Source: CAD feature listing. Evaluate the final solid. Frame: model axes, mm. Give positions to 0.01 mm unless a question says otherwise; leave off trailing zeros. Loops run counter-clockwise (first coordinate to the right, second up) from the corner with the lowest first, then second, coordinate; pieces in that order, holes last. Notation, with made-up numbers: M 74,72 L 90,72 A25 cw 90,97 Z; hole C 17.25,-5.5 d4. An arc over 180 degrees is marked long. Write item = value, one per line.
from build123d import *

# Parameters (mm, degrees)
BOSS_EXTRUDE2_DEPTH = 4
SKETCH2_R           = 3.5
CUT_EXTRUDE1_DEPTH  = 4
SKETCH3_W           = 225
SKETCH3_H           = 150
BOSS_EXTRUDE3_DEPTH = 4


with BuildPart() as part:
    # Sketch1 → Boss-Extrude2 (new body)
    with BuildSketch(Plane(origin=(0, 0, 0), x_dir=(1, 0, 0), z_dir=(0, 1, 0))):
        Polygon((-120, 117), (-120, 150), (-135, 150), (-180, 0), (-135, 0), (0, 0), (45, 0), (0, 150), (-15, 150), (-15, 117), (-30, 117), (-30, 84), (-45, 84), (-45, 51), (-90, 51), (-90, 84), (-105, 84), (-105, 117), align=None)
    extrude(amount=BOSS_EXTRUDE2_DEPTH)

    # Sketch2 → Cut-Extrude1 (cut)
    with BuildSketch(Plane(origin=(0, 4, 0), x_dir=(1, 0, 0), z_dir=(0, 1, 0))):
        with Locations(Location((-127.5, 135, 0), (0, 0, 270))):
            Circle(SKETCH2_R)
        with Locations(Location((-112.5, 102, 0), (0, 0, 270))):
            Circle(SKETCH2_R)
        with Locations(Location((-97.5, 69, 0), (0, 0, 270))):
            Circle(SKETCH2_R)
        with Locations(Location((-78.75, 36, 0), (0, 0, 270))):
            Circle(SKETCH2_R)
        with Locations(Location((-56.25, 36, 0), (0, 0, 90))):
            Circle(SKETCH2_R)
        with Locations(Location((-37.5, 69, 0), (0, 0, 90))):
            Circle(SKETCH2_R)
        with Locations(Location((-22.5, 102, 0), (0, 0, 90))):
            Circle(SKETCH2_R)
        with Locations(Location((-7.5, 135, 0), (0, 0, 90))):
            Circle(SKETCH2_R)
    extrude(amount=-CUT_EXTRUDE1_DEPTH, mode=Mode.SUBTRACT)

    # Sketch3 → Boss-Extrude3 (add)
    with BuildSketch(Plane(origin=(0, 4, 0), x_dir=(1, 0, 0), z_dir=(0, 1, 0))):
        with Locations((-67.5, -75)):
            Rectangle(SKETCH3_W, SKETCH3_H)
    extrude(amount=BOSS_EXTRUDE3_DEPTH)


with BuildPart() as boss_extrude3_kept_piece:
    # of the separate pieces the step leaves, the one the design keeps (boss_extrude3_pieces_kept)
    add(part.part.solids().sort_by_distance((-120, 0, -117))[0])


solid = boss_extrude3_kept_piece.part
1. Cut plane B-B, the plane z = -77. Return the cut outline in (x, y), then the cut area to 3 significant figures.
Derived:
outline = M -156.9,0 L -90,0 L -90,4 L -156.9,4 Z; M -45,0 L 21.9,0 L 21.9,4 L -45,4 Z
area = 535 mm²
2. Cut plane D-D, the plane y = 2.65. Count the separate pieces of the cut face and the enclosed holes in it, then the cut area to 3 significant figures.
Derived:
separate_pieces = 1
enclosed_holes = 8
area = 19,300 mm²
3. Material intervals for probe 1 along X at (y, z) = (2.3, -102); probe 2 along X at (y, z) = (2.75, -69); probe 3 along Z at (x, y) = (-37.5, 2.4), sorted ascending. Write a range as from..to.
Derived:
probe_1 = -149.4..-116, -109..-105, -30..-26, -19..14.4
probe_2 = -159.3..-101, -94..-90, -45..-41, -34..24.3
probe_3 = -84..-72.5, -65.5..0
4. Cut plane A-A, the plane x = -7.5. Return the cut outline in (y, z), then the cut area to 3 significant figures.
Derived:
outline = M 0,-150 L 4,-150 L 4,-138.5 L 0,-138.5 Z; M 0,-131.5 L 4,-131.5 L 4,0 L 0,0 Z
area = 572 mm²
5. Pull-direction query (Z, two-part tool) for faces 1 (the flat face through (-69, 0, -43)), 2 (the cylindrical face through (-8.55, 2.03, -138.34)), 3 (the flat face through (22.8, 2, -74)); classes: +Z half, -Z half, draft (parallel to the pull), parting line (faces both ways), or undercut.
Derived:
face_1 = draft
face_2 = undercut
face_3 = -Z half
6. First-contact query: pin 1 Ø2 at (y, z) = (3, -87.5) entering from +X; pin 2 Ø1.5 at (y, z) = (3, -127.5) entering from -X (3 decimals); pin 3 Ø2 at (y, z) = (3, -126) entering from -X. Flat tips, straight axial feed; report the tip coordinate or a pass-through.
Derived:
pin_1 = 19.05
pin_2 = -141.975
pin_3 = -142.5
7. Cut plane C-C, the plane z = -135. Return the cut outline in (x, y).
Derived:
outline = M -139.5,0 L -131,0 L -131,4 L -139.5,4 Z; M -124,0 L -120,0 L -120,4 L -124,4 Z; M -15,0 L -11,0 L -11,4 L -15,4 Z; M -4,0 L 4.5,0 L 4.5,4 L -4,4 Z
